The drawing under review shows one solid part. Ordinate dimensions are in mm from its lowest x, y, z. Coordinates: 2 decimals unless noted, no trailing zeros. Loops run counter-clockwise (first coordinate to the right, second up) from the corner with the lowest first, then second, coordinate; pieces in that order, holes last. Notation, with made-up numbers: M -37.5,87 L 11.5,87 A29 cw 11.5,123 Z; hole C 27,-32.5 d11. An arc over 180 degrees is marked long. Answer as a JSON object with one key per item and string values. Group by question number.
1. Consider section D-D (x = 0.65). State the section outline as (y, z) points (1 decimal).
2. Consider section C-C (z = 1.5). State the section outline as (x, y) points.
3. Consider section A-A (x = 1.9). State the section outline as (y, z) points.
4. Draft analysis for pull direction Y (two halves, no side actions). For the marked faces 1, 2 and 3, state which applies: +Y half, -Y half, draft (parallel to the pull), parting line (faces both ways), or undercut.
5. To check wall thickness, follow probe 1 along X at (y, z) = (2.75, 7.5) (1 decimal); probe 2 along Y at (x, z) = (2.9, 9); probe 3 along Y at (x, z) = (0.65, 7.5) (1 decimal). State the ranges of each line that lie inside material, in increasing order.
6. Consider section B-B (y = 2.6). State the section outline as (x, z) points (1 decimal).
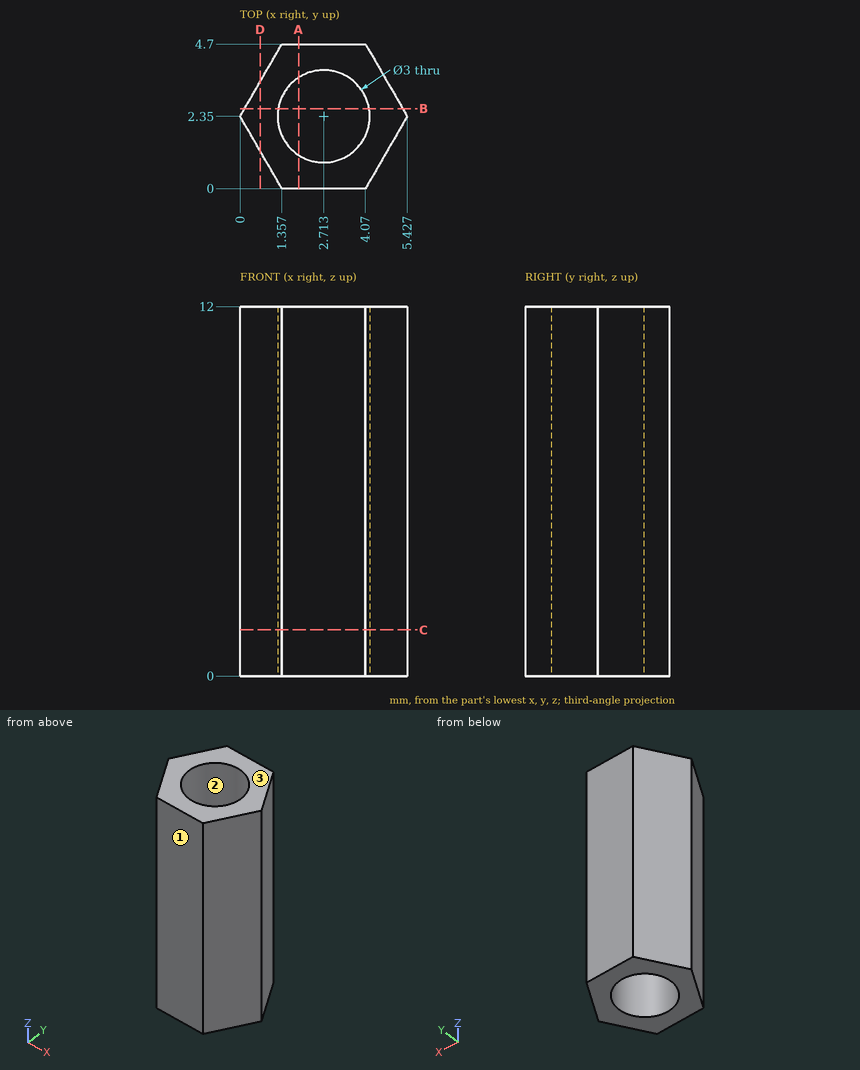
Findings below:
{
 "1": {"outline": "M 1.2,0 L 3.5,0 L 3.5,12 L 1.2,12 Z"},
 "2": {"outline": "M 0,2.35 L 1.36,0 L 4.07,0 L 5.43,2.35 L 4.07,4.7 L 1.36,4.7 Z; hole C 2.71,2.35 d3"},
 "3": {"outline": "M 0,0 L 1.09,0 L 1.09,12 L 0,12 Z; M 3.61,0 L 4.7,0 L 4.7,12 L 3.61,12 Z"},
 "4": {"face 1": "-Y half", "face 2": "undercut", "face 3": "draft"},
 "5": {"probe 1": "x = 0.2 to 1.3, 4.2 to 5.2", "probe 2": "y = 0 to 0.86, 3.84 to 4.7", "probe 3": "y = 1.2 to 3.5"},
 "6": {"outline": "M 0.1,0 L 1.2,0 L 1.2,12 L 0.1,12 Z; M 4.2,0 L 5.3,0 L 5.3,12 L 4.2,12 Z"}
}
